Geometry check sheet. Reference: drawing and pictorial views, mm from the part's lowest x, y, z. Coordinates: 2 decimals unless noted, no trailing zeros. Order: outer loops, then holes, each group sorted by start corner. A loop starts at its lowest first (then second) coordinate and runs counter-clockwise, first axis right, second up. Notation, with made-up numbers: M -25.75,38.5 L 14.25,38.5 A38 cw 14.25,76.5 Z; hole C 17,63.5 d8. An arc over 180 degrees is marked long. Return JSON: item names as keys, results as strings.
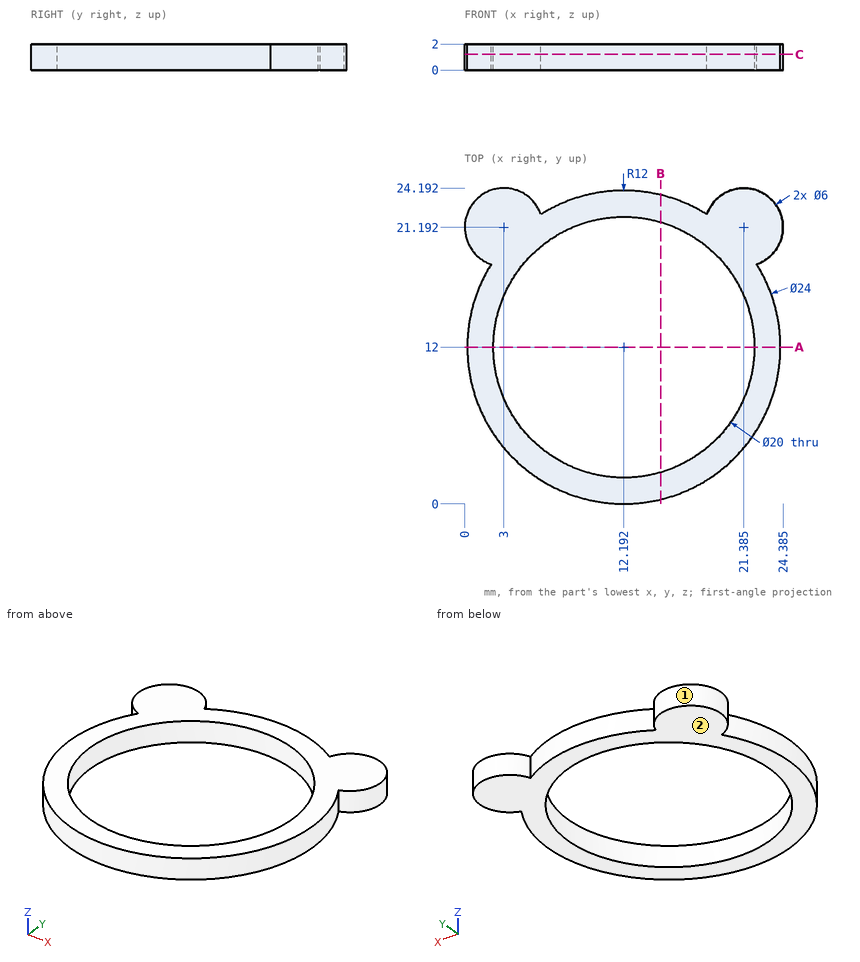
Q1. Cross-section at C-C, the plane z = 1.2. Record the boundary of the cut face in (x, y) (1 decimal).
Values:
{"outline": "M 2,18.4 A12 ccw long 22.4,18.4 A3 ccw long 18.6,22.2 A12 ccw 5.8,22.2 A3 ccw long Z; hole C 12.2,12 d20"}
Q2. Material ranges on line 1 along X through (y, z) = (12, 1.2); line 2 along Y through (x, z) = (12, 0.55); line 3 along X through (y, z) = (14.25, 1.15) (1 decimal), recorded low to high.
Values:
{"line 1": "0.19 to 2.19, 22.19 to 24.19", "line 2": "0 to 2, 22 to 24", "line 3": "0.4 to 2.4, 21.9 to 24"}
Q3. Go/stop test with flat-tipped pins: pin 1 (1 mm diameter, centred on y = 19, z = 1, fed in from -X); pin 2 (1 mm diameter, centred on y = 8, z = 0.5, fed in from -X). Record where each tip stops, or that it passes through.
Values:
{"pin 1": "x = 0.52", "pin 2": "x = 0.71"}
Q4. Cross-section at A-A, the plane y = 12. Record the boundary of the cut face in (x, z).
Values:
{"outline": "M 0.19,0 L 2.19,0 L 2.19,2 L 0.19,2 Z; M 22.19,0 L 24.19,0 L 24.19,2 L 22.19,2 Z"}
Q5. Cross-section at B-B, the plane x = 15. Record the boundary of the cut face in (y, z).
Values:
{"outline": "M 0.33,0 L 2.4,0 L 2.4,2 L 0.33,2 Z; M 21.6,0 L 23.67,0 L 23.67,2 L 21.6,2 Z"}
Q6. Draft check along Y on the marked faces 1 and 2. Enter one of: pulls with the +Y half, pulls with the -Y half, needs draft (parallel to the pull), parting line crosses it, or undercut.
Values:
{"face 1": "undercut", "face 2": "needs draft"}
